```python
from build123d import *

# Parameters (mm, degrees)
EXTRUDE_1_DEPTH     = 2
SKETCH_2_R          = 4.5
SKETCH_2_R_2        = 1.5
CUT_EXTRUDE_1_DEPTH = 91.751684032


with BuildPart() as part:
    # 草图1 → 凸台-拉伸1 (new body)
    with BuildSketch(Plane(origin=(0, 0, 0), x_dir=(1, 0, 0), z_dir=(0, 1, 0))):
        with BuildLine():
            ThreePointArc((3.130434783, 8.438031647), (40, 1.819293264), (76.869565217, 8.438031647))
            ThreePointArc((76.869565217, 8.438031647), (88.32365676, 3.422972121), (83.711340206, -8.199143484))
            ThreePointArc((83.711340206, -8.199143484), (40, -17.63145356), (-3.711340206, -8.199143484))
            ThreePointArc((-3.711340206, -8.199143484), (-8.32365676, 3.422972121), (3.130434783, 8.438031647))
        make_face()
    extrude(amount=EXTRUDE_1_DEPTH)

    # 草图2 → 切除-拉伸1 (cut, through all)
    with BuildSketch(Plane(origin=(0, 2, 0), x_dir=(1, 0, 0), z_dir=(0, 1, 0))):
        with Locations(Location((0, 0, 0), (0, 0, 270))):
            Circle(SKETCH_2_R)
        with Locations(Location((80, 0, 0), (0, 0, 270))):
            Circle(SKETCH_2_R)
        with Locations(Location((7, 0, 0), (0, 0, 270))):
            Circle(SKETCH_2_R_2)
        with Locations(Location((0, -7, 0), (0, 0, 270))):
            Circle(SKETCH_2_R_2)
        with Locations(Location((-7, 0, 0), (0, 0, 270))):
            Circle(SKETCH_2_R_2)
        with Locations(Location((0, 7, 0), (0, 0, 270))):
            Circle(SKETCH_2_R_2)
        with Locations(Location((73, 0, 0), (0, 0, 270))):
            Circle(SKETCH_2_R_2)
        with Locations(Location((80, 7, 0), (0, 0, 270))):
            Circle(SKETCH_2_R_2)
        with Locations(Location((87, 0, 0), (0, 0, 270))):
            Circle(SKETCH_2_R_2)
        with Locations(Location((80, -7, 0), (0, 0, 270))):
            Circle(SKETCH_2_R_2)
    extrude(amount=-CUT_EXTRUDE_1_DEPTH, mode=Mode.SUBTRACT)


solid = part.part
```
Build history of the part. All positions in model axes, mm. Round coordinates to 2 decimals unless told otherwise and drop trailing zeros. Write each loop counter-clockwise with the first axis right and the second up, starting at its lowest first coordinate (ties: lowest second). Pieces come first, ordered by that corner, then holes.
1) Band-saw the part on D-D, the plane z = -6.5. List the corners of the cut face in (x, y), and give its area (3 significant figures).
2) Band-saw the part on C-C, the plane x = 0. List the corners of the cut face in (y, z), and give its area (3 significant figures).
3) Band-saw the part on B-B, the plane y = 0.55. Give the number of separate pieces and of enclosed holes in the cut face, and give its area (3 significant figures).
4) Drill centre lines: probe 1 along X at (y, z) = (1.9, 1.75); probe 2 along X at (y, z) = (0.45, 4); probe 3 along Z at (x, y) = (80.5, 0.5). Where is each one in solid material? Low to high.
5) Pin check, flat tip, straight feed: pin 1 (2.5 mm diameter, centred on x = 0, z = 7, fed in from -Y). Stop position of the tip, or through.
6) Mould opens along Z. For faces 1 (the cylindrical face through (40.63, 0.99, 17.63)), 2 (the cylindrical face through (0.07, 1.01, 5.5)), 3 (the cylindrical face through (-8.395, 0.986, -3.243)) say: +Z half, -Z half, draft (parallel to the pull), parting line (faces both ways), or undercut.
7) Band-saw the part on A-A, the plane z = 0. List the corners of the cut face in (x, y), and give its area (3 significant figures).
Ans:
1. outline: (-6.22, 0) - (-1.41, 0) - (-1.41, 2) - (-6.22, 2) - close; (1.41, 0) - (8.85, 0) - (8.85, 2) - (1.41, 2) - close; (71.15, 0) - (78.59, 0) - (78.59, 2) - (71.15, 2) - close; (81.41, 0) - (86.22, 0) - (86.22, 2) - (81.41, 2) - close
1. area: 49.0 mm2
2. outline: (0, -9) - (2, -9) - (2, -8.5) - (0, -8.5) - close; (0, -5.5) - (2, -5.5) - (2, -4.5) - (0, -4.5) - close; (0, 4.5) - (2, 4.5) - (2, 5.5) - (0, 5.5) - close; (0, 8.5) - (2, 8.5) - (2, 9.79) - (0, 9.79) - close
2. area: 7.59 mm2
3. separate pieces: 1
3. enclosed holes: 10
3. area: 1,630 mm2
4. probe 1: x = -8.83 to -4.15, 4.15 to 75.85, 84.15 to 88.83
4. probe 2: x = -8.06 to -2.06, 2.06 to 77.94, 82.06 to 88.06
4. probe 3: z = -8.99 to -8.41, -5.59 to -4.47, 4.47 to 5.59, 8.41 to 9.59
5. pin 1: passes through
6. face 1: +Z half
6. face 2: undercut
6. face 3: parting line
7. outline: (-9, 0) - (-8.5, 0) - (-8.5, 2) - (-9, 2) - close; (-5.5, 0) - (-4.5, 0) - (-4.5, 2) - (-5.5, 2) - close; (4.5, 0) - (5.5, 0) - (5.5, 2) - (4.5, 2) - close; (8.5, 0) - (71.5, 0) - (71.5, 2) - (8.5, 2) - close; (74.5, 0) - (75.5, 0) - (75.5, 2) - (74.5, 2) - close; (84.5, 0) - (85.5, 0) - (85.5, 2) - (84.5, 2) - close; (88.5, 0) - (89, 0) - (89, 2) - (88.5, 2) - close
7. area: 136 mm2
